Build history of the part. All positions in model axes, mm. A direction names the side the tool comes from. Give positions to 0.01 mm unless a question says otherwise; leave off trailing zeros. Loops run counter-clockwise (first coordinate to the right, second up) from the corner with the lowest first, then second, coordinate; pieces in that order, holes last. Notation, with made-up numbers: M 58,-26 L 71,-26 A11 cw 71,-18 Z; hole C 62,81.5 d11. An arc over 180 degrees is marked long. Answer as a JSON object with one key per item and string values. Group by question number.
1. 3-axis set-ups, long thin cutter, end or side, ignore diameter. For faces 4 (the face through (25, 194, 422.399)), 5 (the face through (25, 376.042, 195)), 6 (the face through (25, 213, 387.601)): which of +Z, -Z, +X, -X, +Y, -Y reach the whole face in a straight line?
2. Slice it at A-A (y = 349.5). List the corners of the cut face in (x, z).
3. Slice it at D-D (z = 593.5). List the corners of the cut face in (x, y).
4. Slice it at B-B (z = 376). List the corners of the cut face in (x, y).
5. Drill centre lines: line 1 along Y through (x, z) = (28.5, 160.5); line 2 along Z through (x, y) = (33, 107.5); line 3 along Y through (x, z) = (34, 666). Where is each one in solid material? Low to high. Write a range as [from, to].
6. Drop flat-ended pins along their axis: pin 1 Ø12 at (x, y) = (20, 96.5) entering from -Z; pin 2 Ø5 at (x, z) = (37.5, 620.5) entering from -Y; pin 3 Ø5 at (x, z) = (25.5, 442.5) entering from -Y. Give the stop position or say it passes through.
7. Slice it at C-C (x = 40). List the corners of the cut face in (y, z), then the cut area to 3 significant figures.
8. Mould opens along Y. For faces 1 (the face through (25.044, 427.373, 620.865)), 2 (the face through (25, 414.142, 213)), 3 (the face through (25, 27, -12.703)) say: released by +Y, released by -Y, zero draft, split by the parting line, or undercut.
from build123d import *

# Parameters (mm, degrees)
F1_DEPTH = 50.8


with BuildPart() as f1:
    # F0 (on Right) → F1 (new body)
    with BuildSketch(Plane.YZ):
        Polygon((7.742018, -9.401204), (7.742018, -12.703204), (45.842018, -12.703204), (45.842018, -9.401204), (45.842018, 384.298796), (376.042018, 384.298796), (376.042018, 4.826), (376.042018, 0), (379.344018, 0), (414.142018, 0), (414.142018, 431.894088), (447.013809, 807.620389), (409.058791, 810.941023), (408.771003, 807.651588), (375.065751, 422.398796), (7.742018, 422.398796), (7.742018, 419.096796), align=None)
        Polygon((42.540018, -9.401204), (11.044018, -9.401204), (11.044018, 419.096796), (374.776864, 419.096796), (378.091477, 419.096796), (379.211095, 431.894088), (412.060438, 807.3638), (443.449104, 804.617647), (410.840018, 431.894088), (410.840018, 3.302), (379.344018, 3.302), (379.344018, 384.298796), (379.344018, 387.600796), (376.042018, 387.600796), (42.540018, 387.600796), (42.540018, 384.298796), align=None, mode=Mode.SUBTRACT)
    extrude(amount=F1_DEPTH)


solid = f1.part
Established:
{
 "1": {"face 4": "+Z, +X, -X, -Y", "face 5": "-Z, +X, -X", "face 6": "+X, -X"},
 "2": {"outline": "M 0,384.3 L 50.8,384.3 L 50.8,387.6 L 0,387.6 Z; M 0,419.1 L 50.8,419.1 L 50.8,422.4 L 0,422.4 Z"},
 "3": {"outline": "M 0,390.04 L 50.8,390.04 L 50.8,393.35 L 0,393.35 Z; M 0,424.98 L 50.8,424.98 L 50.8,428.28 L 0,428.28 Z"},
 "4": {"outline": "M 0,7.74 L 50.8,7.74 L 50.8,11.04 L 0,11.04 Z; M 0,42.54 L 50.8,42.54 L 50.8,45.84 L 0,45.84 Z; M 0,376.04 L 50.8,376.04 L 50.8,379.34 L 0,379.34 Z; M 0,410.84 L 50.8,410.84 L 50.8,414.14 L 0,414.14 Z"},
 "5": {"line 1": "y = [7.74, 11.04], [42.54, 45.84], [376.04, 379.34], [410.84, 414.14]", "line 2": "z = [384.3, 387.6], [419.1, 422.4]", "line 3": "y = [396.38, 399.69], [431.32, 434.62]"},
 "6": {"pin 1": "stops at z = 384.3", "pin 2": "stops at y = 392.18", "pin 3": "stops at y = 376.61"},
 "7": {"outline": "M 7.74,-12.7 L 45.84,-12.7 L 45.84,384.3 L 376.04,384.3 L 376.04,0 L 414.14,0 L 414.14,431.89 L 447.01,807.62 L 409.06,810.94 L 375.07,422.4 L 7.74,422.4 Z; hole M 11.04,-9.4 L 42.54,-9.4 L 42.54,387.6 L 379.34,387.6 L 379.34,3.3 L 410.84,3.3 L 410.84,431.89 L 443.45,804.62 L 412.06,807.36 L 378.09,419.1 L 11.04,419.1 Z", "area": "10,600 mm^2"},
 "8": {"face 1": "undercut", "face 2": "released by +Y", "face 3": "zero draft"}
}
